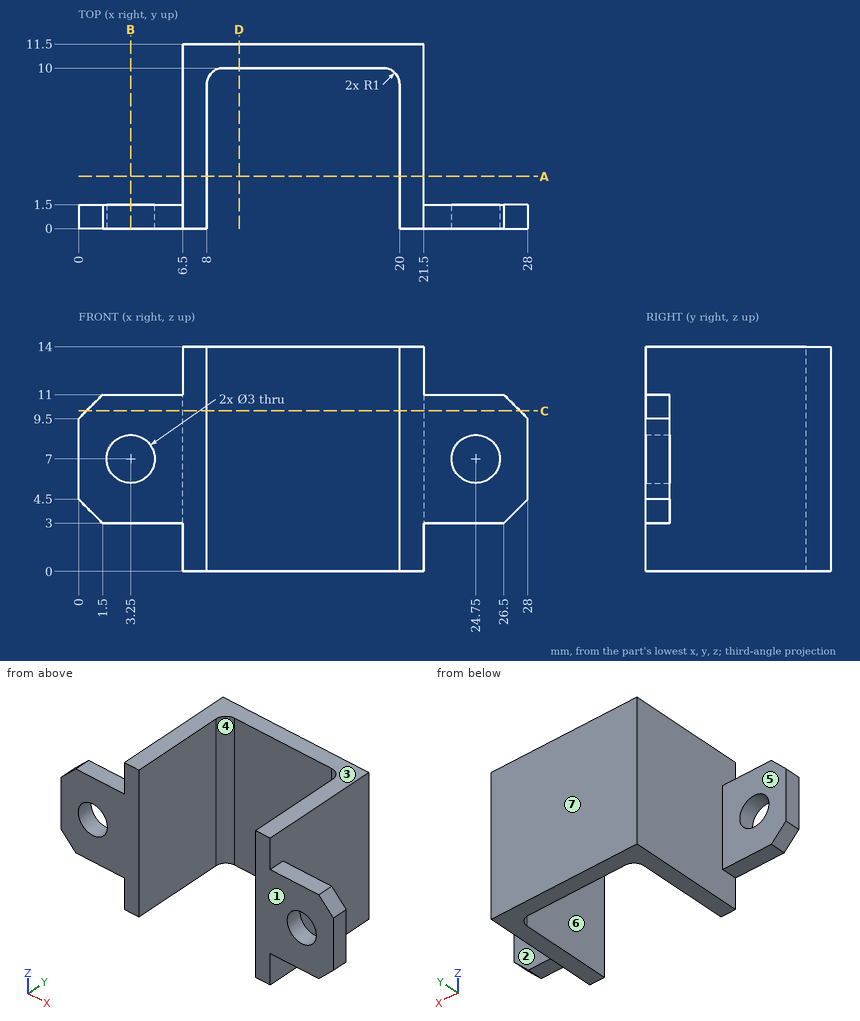
Check sheet for the drawn part. Datum: minimum x, y, z corner. Units: mm. A direction names the side the tool comes from. Round coordinates to 2 decimals unless told otherwise and drop trailing zeros. Write each loop counter-clockwise with the first axis right and the second up, starting at its lowest first coordinate (ties: lowest second). Pieces come first, ordered by that corner, then holes. Notation, with made-up numbers: (24.5, 22.25) -> (61.5, 22.25) arc R21 cw to (61.5, 54.25) -> close; hole circle Ø11 at (-23.5, 70). An arc over 180 degrees is marked (long way). One line per item, written item: value. Start each with the question number.
(1) Go/stop test with flat-tipped pins: pin 1 Ø1.2 at (x, y) = (24.5, 0.5) entering from -Z; pin 2 Ø5 at (y, z) = (8, 12) entering from +X; pin 3 Ø2 at (x, z) = (25.5, 8) entering from +Y. Record where each tip stops, or that it passes through.
(2) Cross-section at D-D, the plane x = 10. Record the cut outline in (y, z).
(3) Draft check along X on the marked faces 6 and 7. Enter one of: +X half, -X half, draft (parallel to the pull), parting line (faces both ways), or undercut.
(4) Scan lines: line 1 (X direction, y = 5, z = 9); line 2 (Z direction, x = 3.25, y = 0.8); line 3 (Y direction, x = 14.75, z = 5.75). Record each from-to range of solid material in increasing order. Write a range as [from, to].
(5) Cross-section at C-C, the plane z = 10. Record the cut outline in (x, y).
(6) Cross-section at A-A, the plane y = 3.25. Record the cut outline in (x, z).
(7) Cross-section at B-B, the plane x = 3.25. Record the cut outline in (y, z).
(8) Access from +Z, -Z, +X, -X, +Y, -Y to the whole of each face (thin tool, end or side, straight path). Record for the marked faces 1, 2, 3, 4 and 5.
Answer:
1. pin 1: z = 3
1. pin 2: x = 21.5
1. pin 3: y = 1.5
2. outline: (10, 0) -> (11.5, 0) -> (11.5, 14) -> (10, 14) -> close
3. face 6: undercut
3. face 7: draft
4. line 1: [6.5, 8], [20, 21.5]
4. line 2: [3, 5.5], [8.5, 11]
4. line 3: [10, 11.5]
5. outline: (0.5, 0) -> (8, 0) -> (8, 9) arc R1 cw to (9, 10) -> (19, 10) arc R1 cw to (20, 9) -> (20, 0) -> (27.5, 0) -> (27.5, 1.5) -> (21.5, 1.5) -> (21.5, 11.5) -> (6.5, 11.5) -> (6.5, 1.5) -> (0.5, 1.5) -> close
6. outline: (6.5, 0) -> (8, 0) -> (8, 14) -> (6.5, 14) -> close; (20, 0) -> (21.5, 0) -> (21.5, 14) -> (20, 14) -> close
7. outline: (0, 3) -> (1.5, 3) -> (1.5, 5.5) -> (0, 5.5) -> close; (0, 8.5) -> (1.5, 8.5) -> (1.5, 11) -> (0, 11) -> close
8. face 1: +Z, -Z, +X, -X, -Y
8. face 2: +Z, -Z, +X, +Y
8. face 3: +Z, +X, -X, +Y, -Y
8. face 4: +Z, -Z, -Y
8. face 5: +Z, -Z, -X, +Y
